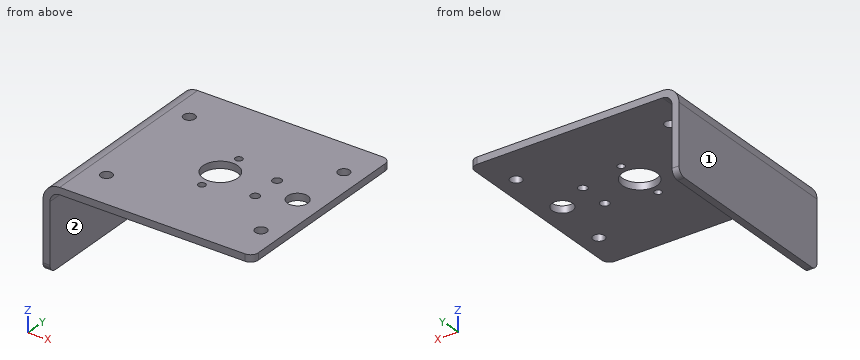
from build123d import *

# Parameters (mm, degrees)
BASE_FLANGE1_DEPTH               = 31.75
FILLET1_R                        = 2.54
F_25_0_1495_DIAMETER_HOLE1_D     = 3.7973
SKETCH10_R                       = 5.715
CUT_EXTRUDE1_DEPTH               = 56.168930099
F_17_64_0_26563_DIAMETER_HOLE1_D = 6.747002
F_3_32_0_09375_DIAMETER_HOLE1_D  = 2.38125
F_32_0_116_DIAMETER_HOLE1_D      = 2.9464


# Sheet-metal steps are written as plain solids
with BuildPart() as part:
    # Sketch3 → Base-Flange1 (new, symmetric)
    with BuildSketch(Plane(origin=(0, 0, 0), x_dir=(-1, 0, 0), z_dir=(0, 1, 0))):
        with BuildLine():
            Line((-33.3375, 0), (30.1625, 0))
            ThreePointArc((30.1625, 0), (32.40756403, -0.92993597), (33.3375, -3.175))
            Line((33.3375, -3.175), (33.3375, -25.4))
            Line((33.3375, -25.4), (35.6235, -25.4))
            Line((35.6235, -25.4), (35.6235, -3.175))
            ThreePointArc((35.6235, -3.175), (34.024010132, 0.686510132), (30.1625, 2.286))
            Line((30.1625, 2.286), (-33.3375, 2.286))
            Line((-33.3375, 2.286), (-33.3375, 0))
        make_face()
    extrude(amount=BASE_FLANGE1_DEPTH, both=True)

    # Fillet1
    fillet1_edges = [part.edges().sort_by_distance(p)[0] for p in [
        (33.3375, 31.75, 1.143),
        (33.3375, -31.75, 1.143),
        (-34.4805, 31.75, -25.4),
        (-34.4805, -31.75, -25.4),
    ]]
    fillet(fillet1_edges, radius=FILLET1_R)

    # #25 (0.1495) Diameter Hole1 (through all)
    with Locations(Plane.XY.offset(2.286)):
        with Locations((-23.8125, 19.05), (26.9875, 19.05), (26.9875, -19.05), (-23.8125, -19.05)):
            Hole(F_25_0_1495_DIAMETER_HOLE1_D / 2)

    # Sketch10 → Cut-Extrude1 (cut, through all)
    with BuildSketch(Plane.XY.offset(2.286)):
        Circle(SKETCH10_R)
    extrude(amount=-CUT_EXTRUDE1_DEPTH, mode=Mode.SUBTRACT)

    # 17/64 (0.26563) Diameter Hole1 (through all)
    with Locations(Plane.XY.offset(2.286)):
        with Locations((25.4, 0)):
            Hole(F_17_64_0_26563_DIAMETER_HOLE1_D / 2)

    # 3/32 (0.09375) Diameter Hole1 (through all)
    with Locations(Plane.XY.offset(2.286)):
        with Locations((0, 8.5), (0, -8.5)):
            Hole(F_3_32_0_09375_DIAMETER_HOLE1_D / 2)

    # #32 (0.116) Diameter Hole1 (through all)
    with Locations(Plane.XY.offset(2.286)):
        with Locations((15.057884182, 5.027499276), (15.057884182, -5.027499276)):
            Hole(F_32_0_116_DIAMETER_HOLE1_D / 2)


solid = part.part
Check sheet for the modelled part. Datum: model origin and axes. Units: mm. Face numbers are marked on the shaded views. A direction names the side the tool comes from. Give positions to 0.01 mm unless a question says otherwise; leave off trailing zeros. Loops run counter-clockwise (first coordinate to the right, second up) from the corner with the lowest first, then second, coordinate; pieces in that order, holes last. Notation, with made-up numbers: M 60,56 L 80,56 A5 cw 80,64 Z; hole C -3.5,46 d2. An arc over 180 degrees is marked long. Answer as a JSON object with one key per item and string values. Group by question number.
Q1. Go/stop test with flat-tipped pins: P1, Ø2.5, axis at x = 15.06, y = 5.03, coming from the -Z side; P2, Ø12, axis at y = -4.5, z = -22, coming from the +X side; P3, Ø4, axis at x = 15.06, y = -5.03, coming from the -Z side. Record where each tip stops, or that it passes through.
Q2. Cross-section at A-A on y = 19.05. Give the number of separate pieces and of enclosed holes in the cut face, then the cut area to 3 significant figures.
Q3. Material ranges on line 1 along Y through (x, z) = (0, 1.7) (3 decimals); line 2 along X through (y, z) = (-29, -14); line 3 along Z through (x, y) = (13, 9), recorded low to high. Write a range as [from, to].
Q4. Access from +Z, -Z, +X, -X, +Y, -Y to the whole of each face (thin tool, end or side, straight path). Record for the marked faces 1 and 2.
Q5. Cross-section at B-B on x = 0. Record the cut outline in (y, z) (3 decimals).
Evaluation:
{
 "1": {"P1": "passes through", "P2": "stops at x = -33.34", "P3": "stops at z = 0"},
 "2": {"separate pieces": "3", "enclosed holes": "0", "area": "194 mm2"},
 "3": {"line 1": "y = [-31.75, -9.691], [-7.309, -5.715], [5.715, 7.309], [9.691, 31.75]", "line 2": "x = [-35.62, -33.34]", "line 3": "z = [0, 2.29]"},
 "4": {"face 1": "+Z, -Z, -X, +Y, -Y", "face 2": "-Z, +X, +Y, -Y"},
 "5": {"outline": "M -31.75,0 L -9.691,0 L -9.691,2.286 L -31.75,2.286 Z; M -7.309,0 L -5.715,0 L -5.715,2.286 L -7.309,2.286 Z; M 5.715,0 L 7.309,0 L 7.309,2.286 L 5.715,2.286 Z; M 9.691,0 L 31.75,0 L 31.75,2.286 L 9.691,2.286 Z"}
}
